The model under review builds one solid part; all positions refer to its coordinate system, in mm. Face numbers are marked on the shaded views. A direction names the side the tool comes from. Coordinates: 2 decimals unless noted, no trailing zeros. Loops run counter-clockwise (first coordinate to the right, second up) from the corner with the lowest first, then second, coordinate; pieces in that order, holes last. Notation, with made-up numbers: M 84,87.5 L 135,87.5 A12 ccw 135,91.5 Z; hole C 48,76 d10. An arc over 180 degrees is marked long. Use one line per item in the form item = value.
```python
from build123d import *

# Parameters (mm, degrees)
F0_R     = 6
F1_DEPTH = 6
F2_DEPTH = 5
F0_R_2   = 3.75
F3_DEPTH = 5.5
F4_DEPTH = 1
F5_R     = 2.55
F6_DEPTH = 1
F7_DEPTH = 3


# Not quite as in the source:
# - a feature names something its author has since deleted; it is built from what else it names


with BuildPart() as f1:
    # F0 (on Front) → F1 (new body, symmetric)
    with BuildSketch(Plane.XZ):
        with BuildLine():
            ThreePointArc((6.7603327111, -4.2776046609), (7.6838356857, -2.2268069417), (8, 0))
            ThreePointArc((8, 0), (-4.6904157598, 6.4807406984), (-2.5, -7.5993420768))
            ThreePointArc((-2.5, -7.5993420768), (0, -8), (2.5, -7.5993420768))
            ThreePointArc((2.5, -7.5993420768), (4.9190370343, -6.3089677963), (6.7603327111, -4.2776046609))
        make_face()
        Circle(F0_R, mode=Mode.SUBTRACT)
        with BuildLine():
            ThreePointArc((2.5, -7.5993420768), (0, -8), (-2.5, -7.5993420768))
            Line((-2.5, -7.5993420768), (-2.5, -10.0993420768))
            Line((-2.5, -10.0993420768), (-2.5, -12.5993420768))
            Line((-2.5, -12.5993420768), (-1.8303241628, -12.5993420768))
            Line((-1.8303241628, -12.5993420768), (-1.25, -12.5993420768))
            Line((-1.25, -12.5993420768), (0, -12.5993420768))
            Line((0, -12.5993420768), (0.85, -12.5993420768))
            Line((0.85, -12.5993420768), (2.5, -12.5993420768))
            Line((2.5, -12.5993420768), (2.5, -7.5993420768))
        make_face()
        Polygon((-2.5, -12.5993420768), (-2.5, -10.0993420768), (-5.25, -12.5993420768), align=None)
        Polygon((2.85, -12.5993420768), (2.5, -12.5993420768), (0.85, -12.5993420768), (0.85, -18.0378015974), (2.85, -18.0378015974), align=None)
        Polygon((8.3499999998, -27.5640810386), (4.4667434126, -20.8380833309), (2.85, -18.0378015974), (0.85, -18.0378015974), (7.8499425387, -30.1621904255), (8.5998597667, -31.4610993824), (20.6315315697, -52.3007943349), (21.192894901, -53.2731147882), (21.8498235115, -54.4109609722), (23.5998091461, -57.4420581792), (25.0328148241, -58.9241157783), (26.1, -58.3079828733), align=None)
        with BuildLine():
            ThreePointArc((41.4522628248, -52.3492529341), (40.2378545238, -51.4173955261), (38.7202154867, -51.6171891785))
            Line((38.7202154867, -51.6171891785), (39.720207278, -53.3492447254))
            Line((39.720207278, -53.3492447254), (41.4522628248, -52.3492529341))
        make_face()
        Polygon((41.4522628248, -52.3492529341), (39.720207278, -53.3492447254), (42.2201867561, -57.6793835925), (43.9522423029, -56.6793918013), align=None)
        Polygon((-1.8303241628, -12.5993420768), (-2.5, -12.5993420768), (-5.25, -12.5993420768), (-5.25, -22.5993420768), (-1.8303241628, -20.5242957716), align=None)
        Polygon((-1.8303241628, -20.5242957716), (-5.25, -22.5993420768), (22.4316151512, -68.2186375255), (25.0052518507, -66.6770817727), (22.4359922626, -62.3876872736), (23.2938711624, -61.8738353559), (19.6969077391, -55.8686830572), (18.9284228965, -54.5804940001), (18.3501014099, -53.6179642353), (5.9549663233, -32.9881126107), (5.1864814807, -31.6999235536), align=None)
        Polygon((34.376104393, -54.107172761), (26.1, -58.3079828733), (25.0328148241, -58.9241157783), (26.4658205021, -60.4061733773), (30.7959593692, -57.9061938992), (32.5280149161, -56.906202108), (38.5902093302, -53.4062308387), (39.720207278, -53.3492447254), (38.7202154867, -51.6171891785), (37.9429287948, -52.2967132374), align=None)
    extrude(amount=F1_DEPTH, both=True)



with BuildPart() as f1b:
    # F0 (on Front) → F1, piece 2 (new body, symmetric)
    with BuildSketch(Plane.XZ):
        Polygon((34.2780005508, -59.937299315), (32.5459450039, -60.9372911063), (30.3808755703, -62.1872808453), (31.3808673616, -63.9193363922), (37.4430617756, -60.4193651228), (36.4430699844, -58.687309576), align=None)
    extrude(amount=F1_DEPTH, both=True)


with BuildPart() as f1_1:
    add(f1.part)

    add(f1b.part)  # F2 merges F1b
    # F0 (on Front) → F2 (join, symmetric)
    with BuildSketch(Plane.XZ):
        Polygon((32.5280149161, -56.906202108), (30.7959593692, -57.9061938992), (32.5459450039, -60.9372911063), (34.2780005508, -59.937299315), align=None)
        Polygon((8.5998597667, -31.4610993824), (7.8499425387, -30.1621904255), (5.1864814807, -31.6999235536), (5.9549663233, -32.9881126107), align=None)
        Polygon((21.192894901, -53.2731147882), (20.6315315697, -52.3007943349), (18.3501014099, -53.6179642353), (18.9284228965, -54.5804940001), align=None)
    extrude(amount=F2_DEPTH, both=True)

    # F0 (on Front) → F3 (join, symmetric)
    with BuildSketch(Plane.XZ):
        Circle(F0_R)
        Circle(F0_R_2, mode=Mode.SUBTRACT)
    extrude(amount=F3_DEPTH, both=True)

    # F0 (on Front) → F4 (join, symmetric)
    with BuildSketch(Plane.XZ):
        with BuildLine():
            Line((5.3327688164, -20.3380833309), (6.7603327111, -4.2776046609))
            ThreePointArc((6.7603327111, -4.2776046609), (4.9190370343, -6.3089677963), (2.5, -7.5993420768))
            Line((2.5, -7.5993420768), (2.5, -12.5993420768))
            Line((2.5, -12.5993420768), (2.85, -12.5993420768))
            Line((2.85, -12.5993420768), (2.85, -18.0378015974))
            Line((2.85, -18.0378015974), (4.4667434126, -20.8380833309))
            Line((4.4667434126, -20.8380833309), (5.3327688164, -20.3380833309))
        make_face()
        Polygon((9.1110238739, -27.1409636232), (8.3499999998, -27.5640810386), (26.1, -58.3079828733), (34.376104393, -54.107172761), align=None)
    extrude(amount=F4_DEPTH, both=True)

    # F5 (on face) → F6 (join)
    with BuildSketch(Plane(origin=(-5.6730972059, 0, -3.2753641989), x_dir=(0, 1, 0), z_dir=(0.8660254038, 0, 0.5))):
        with BuildLine():
            ThreePointArc((0, -28.0461944113), (2.8284271247, -26.8746215361), (4, -24.0461944113))
            ThreePointArc((4, -24.0461944113), (3.1622776602, -21.5967046686), (1, -20.1732110651))
            Line((1, -20.1732110651), (1, -20.279681237))
            Line((1, -20.279681237), (-1, -20.279681237))
            Line((-1, -20.279681237), (-1, -20.1732110651))
            ThreePointArc((-1, -20.1732110651), (-3.9681187851, -24.5502115813), (0, -28.0461944113))
        make_face()
        with Locations((0, -24.0461944113)):
            Circle(F5_R, mode=Mode.SUBTRACT)
    extrude(amount=F6_DEPTH)

    # F5 (on face) → F7 (cut)
    with BuildSketch(Plane(origin=(-5.6730972059, 0, -3.2753641989), x_dir=(0, 1, 0), z_dir=(0.8660254038, 0, 0.5))):
        with Locations((0, -24.0461944113)):
            Circle(F5_R)
    extrude(amount=-F7_DEPTH, mode=Mode.SUBTRACT)


solid = f1_1.part
```
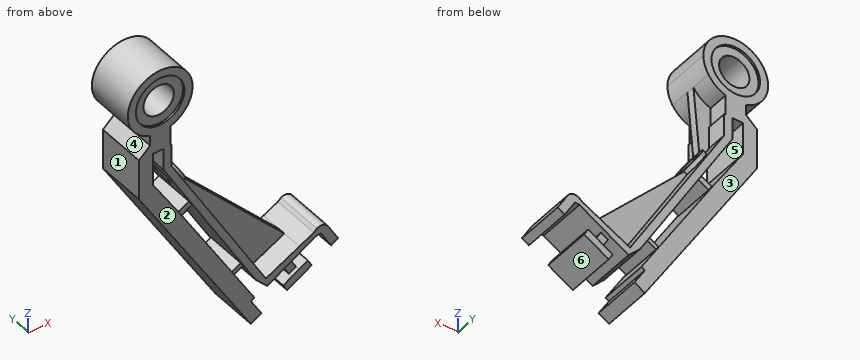
1. Machinability: for the marked faces 1 and 2, which of the approach directions +Z, -Z, +X, -X, +Y, -Y give a long, thin tool a straight path to every point of the face, cutting with its end or side? Answer none if there is none.
Response values:
face_1 = -Z, -X, +Y, -Y
face_2 = +Z, -Z, +X, -X, -Y
2. Add section C-C (x = 0). State the section outline as (y, z) points, then the cut area to 3 significant figures.
Response values:
outline = M -6,-31.25 L 6,-31.25 L 6,-23.44 L -6,-23.44 Z; M -6,-12.6 L 6,-12.6 L 6,-6 L 5.5,-6 L 5.5,-3.75 L -5.5,-3.75 L -5.5,-6 L -6,-6 Z; M -6,6 L -5.5,6 L -5.5,3.75 L 5.5,3.75 L 5.5,6 L 6,6 L 6,8 L -6,8 Z
area = 246 mm^2
3. Add section B-B (z = -47.5). State the section outline as (x, y) points.
Response values:
outline = M 9.86,-6 L 14.67,-6 L 14.67,6 L 9.86,6 Z; M 17.86,-6 L 19.86,-6 L 19.86,-1 L 28.19,-1 L 28.19,1 L 19.86,1 L 19.86,6 L 17.86,6 Z
4. Insertion check: P1, Ø4, axis at y = 1, z = -18.5, coming from the +X side; P2, Ø4, axis at y = 4, z = -16.5, coming from the +X side; P3, Ø1.5, axis at y = -1, z = -40.5, coming from the -X side. Each pin has a flat end and moves straight along its axis. Give the tip position at first contact, or say it passes through.
Response values:
P1 = 5.67
P2 = 3.12
P3 = 5.16
5. Add section A-A (x = 14). State the section outline as (y, z) points, then the cut area to 3 significant figures.
Response values:
outline = M -6,-54.32 L 6,-54.32 L 6,-46.38 L -6,-46.38 Z; M -6,-40.81 L 6,-40.81 L 6,-37.35 L 1,-37.35 L 1,-32.36 L -1,-32.36 L -1,-37.35 L -6,-37.35 Z
area = 147 mm^2
6. Wall thickness on line 1 along Z through (x, y) = (0, -5.8); line 2 along Z through (x, y) = (1, 4.25); line 3 along X through (y, z) = (0.5, -53): over which ranges is each line inside the solid? List them lowest first. Write a range as from..to.
Response values:
line_1 = -31.25..-23.44, -12.6..-6, 6..8
line_2 = -32.9..-25.03, -18.3..-3.61, 3.61..7.94
line_3 = 13.2..17.98, 19.42..33.34, 36.56..41.83
7. The part is to be moulded in two halves that separate along Z. For the marked faces 3, 4, 5 and 6, say which applies: pulls with the +Z half, pulls with the -Z half, needs draft (parallel to the pull), parting line crosses it, or undercut.
Response values:
face_3 = needs draft
face_4 = undercut
face_5 = undercut
face_6 = pulls with the -Z half
